```python
from build123d import *

# Parameters (mm, degrees)
F0_R      = 12.5
F1_DEPTH  = 22
F2_R      = 12.2
F3_DEPTH  = 30.8
F4_R      = 3.5
F5_DEPTH  = 2.5
F6_R      = 2
F7_DEPTH  = 22
F9_DEPTH  = 17.5
F10_R     = 1.5
F11_DEPTH = 4


with BuildPart() as f1:
    # F0 (on Top) → F1 (new body)
    with BuildSketch(Plane.XY):
        Circle(F0_R)
    extrude(amount=-F1_DEPTH)

    # F2 (on face) → F3 (join)
    with BuildSketch(Plane(origin=(0, 0, -22), x_dir=(1, 0, 0), z_dir=(0, 0, -1))):
        Circle(F2_R)
    extrude(amount=F3_DEPTH)

    # F4 (on face) → F5 (join)
    with BuildSketch(Plane.XY):
        Circle(F4_R)
    extrude(amount=F5_DEPTH)

    # F6 (on face) → F7 (join)
    with BuildSketch(Plane.XY):
        Circle(F6_R)
    extrude(amount=F7_DEPTH)

    # F8 (on face) → F9 (cut)
    with BuildSketch(Plane.XY.offset(22)):
        with BuildLine():
            Line((1.322876, -1.5), (-1.322876, -1.5))
            ThreePointArc((-1.322876, -1.5), (0, -2), (1.322876, -1.5))
        make_face()
    extrude(amount=-F9_DEPTH, mode=Mode.SUBTRACT)

    # F10 (on face) → F11 (cut)
    with BuildSketch(Plane.XY):
        with Locations((-8.5, 0)):
            Circle(F10_R)
        with Locations((8.5, 0)):
            Circle(F10_R)
    extrude(amount=-F11_DEPTH, mode=Mode.SUBTRACT)


solid = f1.part
```
Geometry check sheet. Reference: the model listing, model coordinates, mm. A direction names the side the tool comes from. Round coordinates to 2 decimals unless told otherwise and drop trailing zeros. Loops run counter-clockwise (first coordinate to the right, second up) from the corner with the lowest first, then second, coordinate; pieces in that order, holes last. Notation, with made-up numbers: M 14.25,2.25 L 27.25,2.25 A20 ccw 27.25,26.25 Z; hole C -34,63 d4. An arc over 180 degrees is marked long. Return JSON: item names as keys, results as strings. Group by question number.
(1) Scan lines: line 1 along Z through (x, y) = (-8, 4.5); line 2 along Z through (x, y) = (-7.5, -9.75); line 3 along X through (y, z) = (7, -34). Record each from-to range of solid material in increasing order. Write a range as [from, to].
(2) Section check D-D, the plane x = -8.5. Enter the section's corners in (y, z), and give its area (3 significant figures).
(3) Section check A-A, the plane y = 0. Enter the section's corners in (x, z).
(4) Section check B-B, the plane x = 0. Enter the section's corners in (y, z), and give its area (3 significant figures).
(5) Mould release check, pull along X, two halves, no side actions. Record for faces 1 (the face through (3, -3, 0)), 2 (the face through (7.3, -0.9, -2)), 3 (the face through (11.923, 3.755, -10.846)): pulls with the +X half, pulls with the -X half, needs draft (parallel to the pull), parting line crosses it, or undercut.
(6) Go/stop test with flat-tipped pins: pin 1 (0.9 mm diameter, centred on x = -9, y = 0, fed in from +Z); pin 2 (5 mm diameter, centred on x = -7.5, z = -20.5, fed in from +Y); pin 3 (0.8 mm diameter, centred on x = -0.5, z = 14, fed in from -Y). Record where each tip stops, or that it passes through.
(7) Section check C-C, the plane z = -13. Enter the section's corners in (x, y).
(8) Set-up check for faces 4 (the face through (0, -1.5, 13)), 5 (the face through (2, -2, 2.5)), 6 (the face through (-12.19, -0.54, -37.18)): record each of +Z, -Z, +X, -X, +Y, -Y from which the full face is reachable in a straight line by a thin tool's end or side.
Data:
{
 "1": {"line 1": "[-52.8, 0]", "line 2": "[-22, 0]", "line 3": "[-9.99, 9.99]"},
 "2": {"outline": "M -9.17,-22 L -8.75,-22 L -8.75,-52.8 L 8.75,-52.8 L 8.75,-22 L 9.17,-22 L 9.17,0 L 1.5,0 L 1.5,-4 L -1.5,-4 L -1.5,0 L -9.17,0 Z", "area": "930 mm²"},
 "3": {"outline": "M -12.5,-22 L -12.2,-22 L -12.2,-52.8 L 12.2,-52.8 L 12.2,-22 L 12.5,-22 L 12.5,0 L 10,0 L 10,-4 L 7,-4 L 7,0 L 3.5,0 L 3.5,2.5 L 2,2.5 L 2,22 L -2,22 L -2,2.5 L -3.5,2.5 L -3.5,0 L -7,0 L -7,-4 L -10,-4 L -10,0 L -12.5,0 Z"},
 "4": {"outline": "M -12.5,-22 L -12.2,-22 L -12.2,-52.8 L 12.2,-52.8 L 12.2,-22 L 12.5,-22 L 12.5,0 L 3.5,0 L 3.5,2.5 L 2,2.5 L 2,22 L -1.5,22 L -1.5,4.5 L -2,4.5 L -2,2.5 L -3.5,2.5 L -3.5,0 L -12.5,0 Z", "area": "1,390 mm²"},
 "5": {"face 1": "needs draft", "face 2": "undercut", "face 3": "parting line crosses it"},
 "6": {"pin 1": "z = -4", "pin 2": "y = 11.46", "pin 3": "y = -1.5"},
 "7": {"outline": "C 0,0 d25"},
 "8": {"face 4": "+Z, +X, -X, -Y", "face 5": "+Z", "face 6": "-Z"}
}
